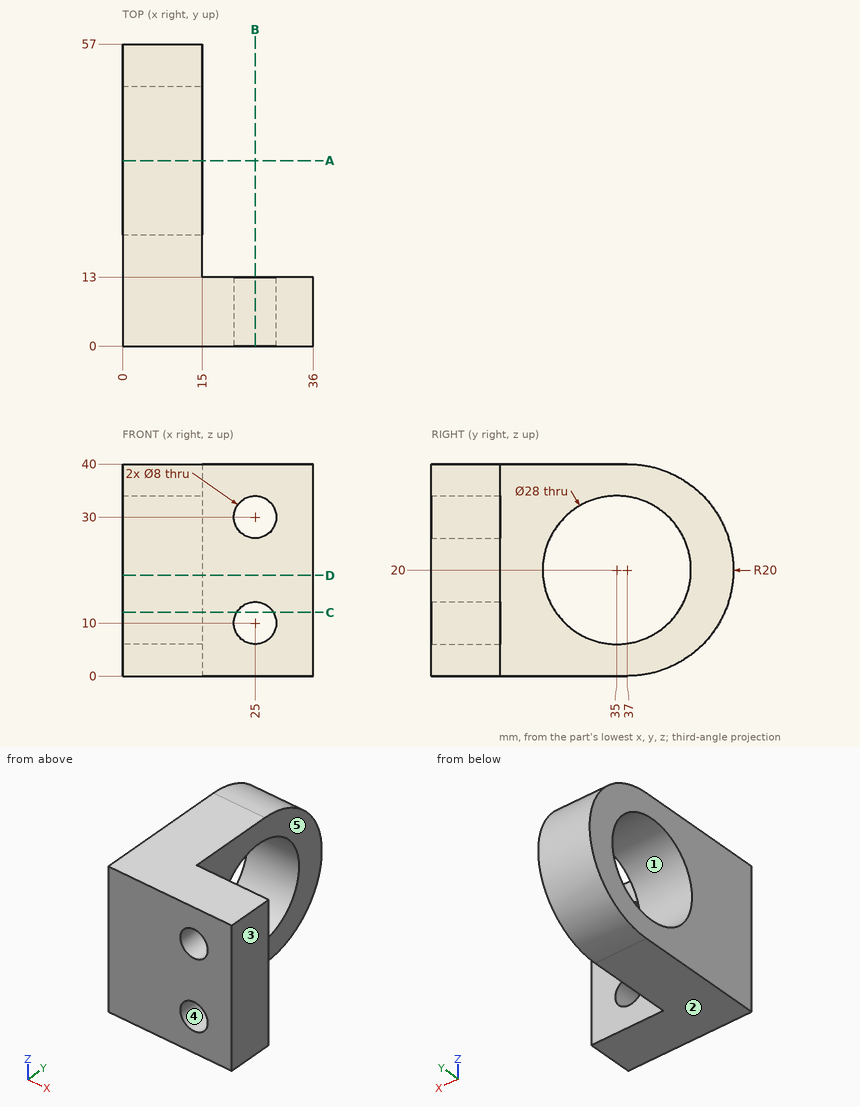
Part print with two shaded views. Sizes in mm from the minimum x, y, z corner. A direction names the side the tool comes from. Round coordinates to 2 decimals unless told otherwise and drop trailing zeros. Loops run counter-clockwise (first coordinate to the right, second up) from the corner with the lowest first, then second, coordinate; pieces in that order, holes last. Notation, with made-up numbers: M 40.5,71.25 L 98.5,71.25 A29 cw 98.5,94.25 Z; hole C -35.75,16.25 d10. An arc over 180 degrees is marked long. Return JSON: item names as keys, results as strings. Group by question number.
(1) Wall check: probe 1 along Z at (x, y) = (25, 7); probe 2 along X at (y, z) = (49.5, 35.5); probe 3 along Y at (x, z) = (5, 22). Give the ranges that are in metal, low to high. Write a range as [from, to].
(2) Saw through at B-B, the plane x = 25. List the corners of the cut face in (y, z).
(3) Mould opens along Z. For the marked faces 1, 2 and 3 say: +Z half, -Z half, draft (parallel to the pull), parting line (faces both ways), or undercut.
(4) Saw through at D-D, the plane z = 19. List the corners of the cut face in (x, y).
(5) Tool access for the marked faces 4 and 5: list every direction of +Z, -Z, +X, -X, +Y, -Y with a clear straight run to the whole face (end or side of a thin tool).
(6) Drop flat-ended pins along their axis: P1, Ø5, axis at x = 19, y = 17.5, coming from the +Z side; P2, Ø3, axis at x = 23, z = 13.5, coming from the +Y side; P3, Ø5, axis at x = 9.5, z = 16, coming from the +Y side. Give the stop position or say it passes through.
(7) Saw through at A-A, the plane y = 35. List the corners of the cut face in (x, z).
(8) Saw through at C-C, the plane z = 12. List the corners of the cut face in (x, y), and give its area (3 significant figures).
Answer list:
{
 "1": {"probe 1": "[0, 6], [14, 26], [34, 40]", "probe 2": "[0, 15]", "probe 3": "[0, 21.14], [48.86, 56.9]"},
 "2": {"outline": "M 0,0 L 13,0 L 13,6 L 0,6 Z; M 0,14 L 13,14 L 13,26 L 0,26 Z; M 0,34 L 13,34 L 13,40 L 0,40 Z"},
 "3": {"face 1": "undercut", "face 2": "-Z half", "face 3": "draft"},
 "4": {"outline": "M 0,0 L 36,0 L 36,13 L 15,13 L 15,21.04 L 0,21.04 Z; M 0,48.96 L 15,48.96 L 15,56.97 L 0,56.97 Z"},
 "5": {"face 4": "+Y, -Y", "face 5": "+Z, -Z, +X, +Y"},
 "6": {"P1": "through", "P2": "y = 13", "P3": "y = 56.94"},
 "7": {"outline": "M 0,0 L 15,0 L 15,6 L 0,6 Z; M 0,34 L 15,34 L 15,40 L 0,40 Z"},
 "8": {"outline": "M 0,0 L 21.54,0 L 21.54,13 L 15,13 L 15,23.51 L 0,23.51 Z; M 0,46.49 L 15,46.49 L 15,55.33 L 0,55.33 Z; M 28.46,0 L 36,0 L 36,13 L 28.46,13 Z", "area": "668 mm2"}
}
